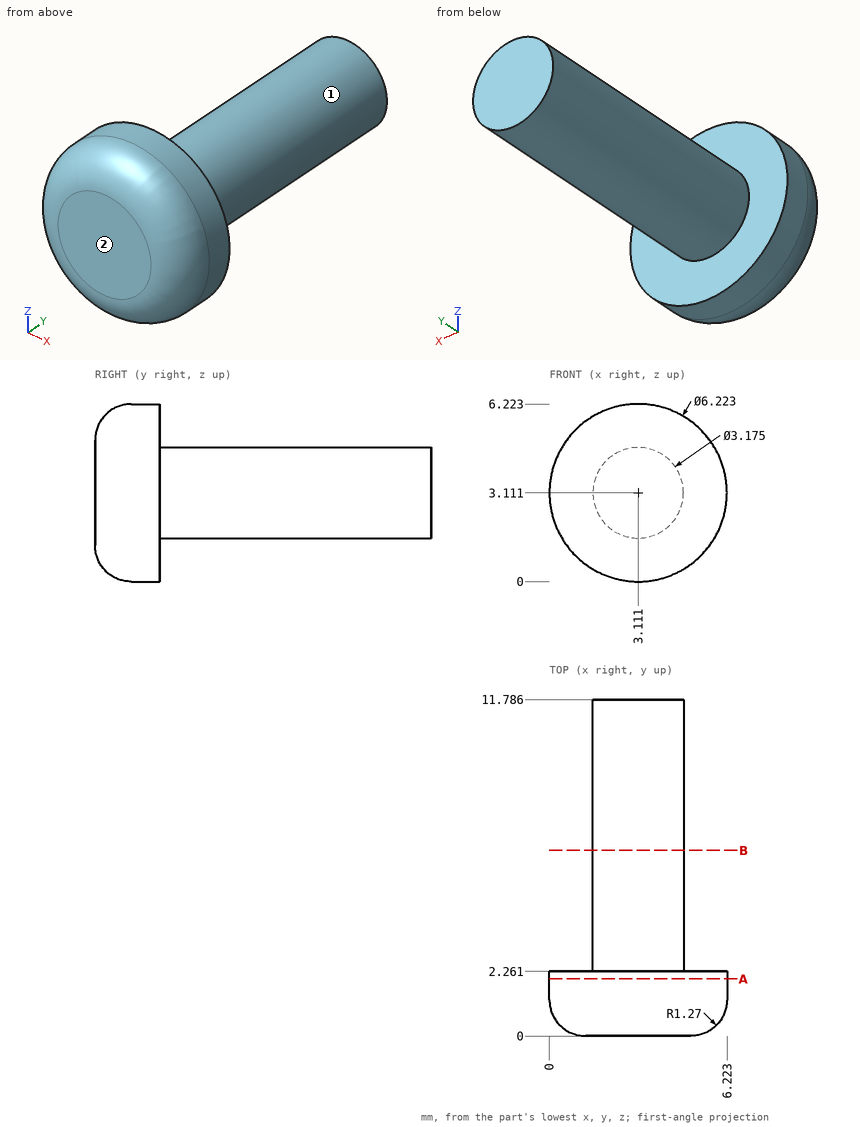
Can you work these out from the drawing? Everything is in mm from the part's minimum corner. A direction names the side the tool comes from. Coordinates: 2 decimals unless noted, no trailing zeros. Loops run counter-clockwise (first coordinate to the right, second up) from the corner with the lowest first, then second, coordinate; pieces in that order, holes last.
1) Imagine slicing it at A-A on y = 2. List the corners of the cut face in (x, z) for me, plus the area to 3 significant figures.
2) I need wall thicknesses on probe 1 along Y at (x, z) = (4, 4.5); probe 2 along X at (y, z) = (1.5, 3.25); probe 3 along Y at (x, z) = (4.25, 0.5) (1 decimal). Which ranges of each line are inside material? Lowest first, please.
3) Which directions (+Z, -Z, +X, -X, +Y, -Y) give clear straight access to the entire face, cutting with the end or side of a thin tool? Please do the marked faces 1 and 2.
4) Imagine slicing it at B-B on y = 6.5. List the corners of the cut face in (x, z) for me (1 decimal).
5) For pin 1 (2 mm diameter, centred on y = 10.5, z = 4, fed in from +X); pin 2 (2 mm diameter, centred on x = 1, y = 7, fed in from -Z), each with a flat end and sliding along its axis, tell me the tip position at first contact or that it passes through.
Completed:
1. outline: circle Ø6.22 at (3.11, 3.11)
1. area: 30.4 mm2
2. probe 1: y = 0 to 2.26
2. probe 2: x = 0 to 6.22
2. probe 3: y = 0.5 to 2.3
3. face 1: +Y
3. face 2: +Z, -Z, +X, -X, -Y
4. outline: circle Ø3.2 at (3.1, 3.1)
5. pin 1: stops at x = 4.7
5. pin 2: stops at z = 1.98
